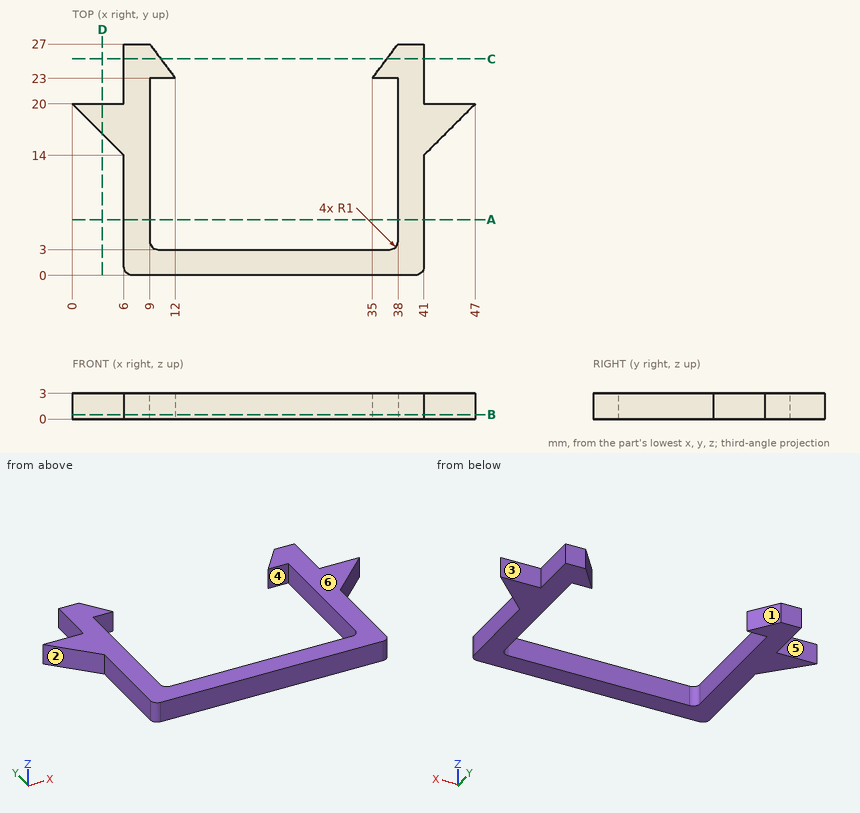
Input: dimensioned drawing with shaded views. Units: mm. Origin: part minimum x, y, z. A direction names the side the tool comes from. Coordinates: 2 decimals unless noted, no trailing zeros. Loops run counter-clockwise (first coordinate to the right, second up) from the corner with the lowest first, then second, coordinate; pieces in that order, holes last. Notation, with made-up numbers: (-6, 20.25) -> (1, 20.25) arc R30 cw to (1, 45.25) -> close; hole circle Ø11 at (67.25, 35). An arc over 180 degrees is marked (long way). Use a Markdown table: item, result. Add a question column.
(1) Line query: line 1 along X through (y, z) = (9.5, 0.5); line 2 along Y through (x, z) = (16.5, 1.2); line 3 along X through (y, z) = (1.5, 0.15). Output: solid intervals per line, ascending.
(2) Pin query (flat end, axial travel): pin 1 Ø1.5 at (y, z) = (10.5, 1.5) entering from +X; pin 2 Ø1.5 at (y, z) = (25, 1) entering from -X; pin 3 Ø4 at (x, y) = (12, 16) entering from -Z; pin 4 Ø0.9 at (x, z) = (22, 1) entering from +Y. Return the tip coordinate at first contact, or that it passes through.
(3) Section query D-D, the plane x = 3.5. Return loops of the section in (y, z).
(4) Section query C-C, the plane y = 25.25. Return loops of the section in (x, z), plus the area to 3 significant figures.
(5) Section query B-B, the plane z = 0.5. Return loops of the section in (x, y).
(6) Section query A-A, the plane y = 6.5. Return loops of the section in (x, z), plus the area to 3 significant figures.
(7) Access query for the marked faces 4, 5 and 6. Directions: +Z, -Z, +X, -X, +Y, -Y. A direction counts if a zero-diameter tool reaches every point of the face in a straight line with its end or side. Return the directions, or none.
(8) Mould query, pull axis X, two halves, no side actions, for the marked faces 1, 2 and 3. Classes: pulls with the +X half, pulls with the -X half, needs draft (parallel to the pull), parting line crosses it, or undercut.
Answer:
| question | item | result |
|---|---|---|
| 1 | line 1 | x = 6 to 9, 38 to 41 |
| 1 | line 2 | y = 0 to 3 |
| 1 | line 3 | x = 6 to 41 |
| 2 | pin 1 | stops at x = 41 |
| 2 | pin 2 | stops at x = 6 |
| 2 | pin 3 | passes through |
| 2 | pin 4 | stops at y = 3 |
| 3 | outline | (16.5, 0) -> (20, 0) -> (20, 3) -> (16.5, 3) -> close |
| 4 | outline | (6, 0) -> (10.31, 0) -> (10.31, 3) -> (6, 3) -> close; (36.69, 0) -> (41, 0) -> (41, 3) -> (36.69, 3) -> close |
| 4 | area | 25.9 mm^2 |
| 5 | outline | (0, 20) -> (6, 14) -> (6, 1) arc R1 ccw to (7, 0) -> (40, 0) arc R1 ccw to (41, 1) -> (41, 14) -> (47, 20) -> (41, 20) -> (41, 27) -> (38, 27) -> (35, 23) -> (38, 23) -> (38, 4) arc R1 cw to (37, 3) -> (10, 3) arc R1 cw to (9, 4) -> (9, 23) -> (12, 23) -> (9, 27) -> (6, 27) -> (6, 20) -> close |
| 6 | outline | (6, 0) -> (9, 0) -> (9, 3) -> (6, 3) -> close; (38, 0) -> (41, 0) -> (41, 3) -> (38, 3) -> close |
| 6 | area | 18.0 mm^2 |
| 7 | face 4 | +Z, -Z |
| 7 | face 5 | +Z, -Z, -X, +Y |
| 7 | face 6 | +Z, +X, -X, +Y, -Y |
| 8 | face 1 | undercut |
| 8 | face 2 | pulls with the -X half |
| 8 | face 3 | needs draft |
